```python
from build123d import *

# Parameters (mm, degrees)
IZIM1_W                     = 65
IZIM1_H                     = 42
Y_KSEKLIK_EKSTR_ZYON1_DEPTH = 80
IZIM3_R                     = 20
KES_EKSTR_ZYON1_DEPTH       = 81
KES_EKSTR_ZYON2_DEPTH       = 41
KES_EKSTR_ZYON5_DEPTH       = 65
KES_EKSTR_ZYON6_DEPTH       = 156
KES_EKSTR_ZYON6_DEPTH_BACK  = 1


with BuildPart() as part:
    # Çizim1 → Yükseklik-Ekstrüzyon1 (new body)
    with BuildSketch(Plane.XY):
        with BuildLine():
            Line((-120, -72), (-100, -72))
            Line((-100, -72), (0, -72))
            Line((0, -72), (20, -72))
            Line((20, -72), (20, -20))
            ThreePointArc((20, -20), (14.142135624, -5.857864376), (0, 0))
            Line((0, 0), (-17.5, 0))
            Line((-17.5, 0), (-17.5, -42))
            Line((-17.5, -42), (-82.5, -42))
            Line((-82.5, -42), (-82.5, 0))
            Line((-82.5, 0), (-100, 0))
            ThreePointArc((-100, 0), (-114.142135624, -5.857864376), (-120, -20))
            Line((-120, -20), (-120, -72))
        make_face()
        with Locations((-50, -21)):
            Rectangle(IZIM1_W, IZIM1_H)
    extrude(amount=Y_KSEKLIK_EKSTR_ZYON1_DEPTH)

    # Çizim3 → Kes-Ekstrüzyon1 (cut, through all)
    with BuildSketch(Plane.XY.offset(80)):
        with Locations((-50, 0)):
            Circle(IZIM3_R)
    extrude(amount=-KES_EKSTR_ZYON1_DEPTH, mode=Mode.SUBTRACT)

    # Çizim4 → Kes-Ekstrüzyon2 (cut)
    with BuildSketch(Plane.XY.offset(80)):
        with BuildLine():
            ThreePointArc((-30, 0), (-50, -20), (-70, 0))
            Line((-70, 0), (-82.5, 0))
            Line((-82.5, 0), (-82.5, -42))
            Line((-82.5, -42), (-17.5, -42))
            Line((-17.5, -42), (-17.5, 0))
            Line((-17.5, 0), (-30, 0))
        make_face()
    extrude(amount=-KES_EKSTR_ZYON2_DEPTH, mode=Mode.SUBTRACT)

    # Çizim5 → Kes-Ekstrüzyon5 (cut)
    with BuildSketch(Plane.XY.offset(80)):
        with BuildLine():
            Line((-120, -20), (-120, -72))
            Line((-120, -72), (-98, -72))
            Line((-98, -72), (-98, -54))
            ThreePointArc((-98, -54), (-94.485281374, -45.514718626), (-86, -42))
            Line((-86, -42), (-82.5, -42))
            Line((-82.5, -42), (-82.5, 0))
            Line((-82.5, 0), (-100, 0))
            ThreePointArc((-100, 0), (-114.142135624, -5.857864376), (-120, -20))
        make_face()
        with BuildLine():
            Line((-2, -54), (-2, -72))
            Line((-2, -72), (20, -72))
            Line((20, -72), (20, -20))
            ThreePointArc((20, -20), (14.142135624, -5.857864376), (0, 0))
            Line((0, 0), (-17.5, 0))
            Line((-17.5, 0), (-17.5, -42))
            Line((-17.5, -42), (-14, -42))
            ThreePointArc((-14, -42), (-5.514718626, -45.514718626), (-2, -54))
        make_face()
        Polygon((-85.547005384, -52), (-74, -72), (-26, -72), (-14.452994616, -52), align=None)
    extrude(amount=-KES_EKSTR_ZYON5_DEPTH, mode=Mode.SUBTRACT)

    # Çizim16 → Kes-Ekstrüzyon6 (cut, two sides)
    with BuildSketch(Plane.XY) as kes_ekstr_zyon6_sk:
        Polygon((-74, -72), (-85.547005384, -52), (-14.452994616, -52), (-26, -72), align=None)
    extrude(amount=KES_EKSTR_ZYON6_DEPTH, mode=Mode.SUBTRACT)
    extrude(kes_ekstr_zyon6_sk.sketch, amount=-KES_EKSTR_ZYON6_DEPTH_BACK, mode=Mode.SUBTRACT)


solid = part.part
```
Can you work these out from the model? Positions are in its coordinate system, mm. A direction names the side the tool comes from. Coordinates: 2 decimals unless noted, no trailing zeros. Order: outer loops, then holes, each group sorted by start corner. A loop starts at its lowest first (then second) coordinate and runs counter-clockwise, first axis right, second up. Notation, with made-up numbers: (39.25, 44) - (65.25, 44) arc R20 cw to (65.25, 72) - close; hole circle Ø7 at (4, 38.5). An arc over 180 degrees is marked (long way). Answer in a Markdown table with one row per item.
1. For faces 1 (the cylindrical face through (-113.986, -5.703, 7.395)), 2 (the flat face through (-82.5, -21, 27)), 3 (the flat face through (-50, -25, 39)), 4 (the cylindrical face through (-5.61, -45.42, 47.96)), 5 (the flat face through (-98, -63, 48)), which set-ups out of +Z, -Z, +X, -X, +Y, -Y let a thin tool reach every point of the face, with its end or its side?
Reply:
| item | result |
|---|---|
| face 1 | +Z, -Z, -X, +Y |
| face 2 | +Z, -X, +Y |
| face 3 | +Z, +X, -X, +Y |
| face 4 | +Z, +X, +Y |
| face 5 | +Z, -X, +Y, -Y |
2. Suppose I cut it at A-A (z = 49). Please give me the cut outline in (x, y), and give its area (3 significant figures).
Reply:
| item | result |
|---|---|
| outline | (-98, -72) - (-74, -72) - (-85.55, -52) - (-14.45, -52) - (-26, -72) - (-2, -72) - (-2, -54) arc R12 ccw to (-14, -42) - (-86, -42) arc R12 ccw to (-98, -54) - close |
| area | 1,630 mm^2 |
3. If I drill on line 1 along Z through (x, y) = (-3, -29); line 2 along X through (y, z) = (-53, 10); line 3 along X through (y, z) = (-8.5, 11.5), over which ranges is the centre line in solid material (lowest first)?
Reply:
| item | result |
|---|---|
| line 1 | z = 0 to 15 |
| line 2 | x = -120 to -84.97, -15.03 to 20 |
| line 3 | x = -116.36 to -68.1, -31.9 to 16.36 |
4. Suppose I cut it at C-C (x = -28.5). Please give me the cut outline in (y, z), and give its area (3 significant figures).
Reply:
| item | result |
|---|---|
| outline | (-52, 0) - (0, 0) - (0, 39) - (-42, 39) - (-42, 80) - (-52, 80) - close |
| area | 2,440 mm^2 |
5. For pin 1 (11 mm diameter, centred on x = 5, y = -38.5, fed in from +Z); pin 2 (21.5 mm diameter, centred on x = -67, z = 26.5, fed in from -Y); pin 3 (1.5 mm diameter, centred on y = -59, z = 69.5, fed in from +X); pin 4 (4 mm diameter, centred on x = -70.5, z = 70.5, fed in from -Y), each with a flat end and sliding along its axis, tell me the tip position at first contact or that it passes through.
Reply:
| item | result |
|---|---|
| pin 1 | stops at z = 15 |
| pin 2 | stops at y = -72 |
| pin 3 | stops at x = -2 |
| pin 4 | stops at y = -52 |
6. Suppose I cut it at D-D (y = -8). Please give me the cut outline in (x, z), and give its area (3 significant figures).
Reply:
| item | result |
|---|---|
| outline | (-116, 0) - (-68.33, 0) - (-68.33, 39) - (-82.5, 39) - (-82.5, 15) - (-116, 15) - close; (-31.67, 0) - (16, 0) - (16, 15) - (-17.5, 15) - (-17.5, 39) - (-31.67, 39) - close |
| area | 2,110 mm^2 |
7. Suppose I cut it at B-B (y = -21.5). Please give me the cut outline in (x, z), and give its area (3 significant figures).
Reply:
| item | result |
|---|---|
| outline | (-120, 0) - (20, 0) - (20, 15) - (-17.5, 15) - (-17.5, 39) - (-82.5, 39) - (-82.5, 15) - (-120, 15) - close |
| area | 3,660 mm^2 |
8. If we mould it in two halves opening along Y, with no side actions, what happens to faces 6 (the flat face through (-2, -63, 48)), 7 (the flat face through (-20.146, -61.86, 39.44)), 8 (the cylindrical face through (-50, -20, 20)), 9 (the flat face through (-79.693, -62.14, 39.44))? For each: pulls with the +Y half, pulls with the -Y half, needs draft (parallel to the pull), parting line crosses it, or undercut.
Reply:
| item | result |
|---|---|
| face 6 | needs draft |
| face 7 | undercut |
| face 8 | pulls with the +Y half |
| face 9 | undercut |
